Can you work these out from the model? Positions are in its coordinate system, mm. Face numbers are marked on the shaded views. A direction names the side the tool comes from. Give positions to 0.01 mm unless a question says otherwise; leave off trailing zeros. Loops run counter-clockwise (first coordinate to the right, second up) from the corner with the lowest first, then second, coordinate; pieces in that order, holes last. Notation, with made-up numbers: (47, 57) - (89, 57) arc R12 cw to (89, 72) - close; hole circle Ø5 at (-10.75, 67). An arc over 180 degrees is marked (long way). Answer as a JSON object with one key per item and string values.
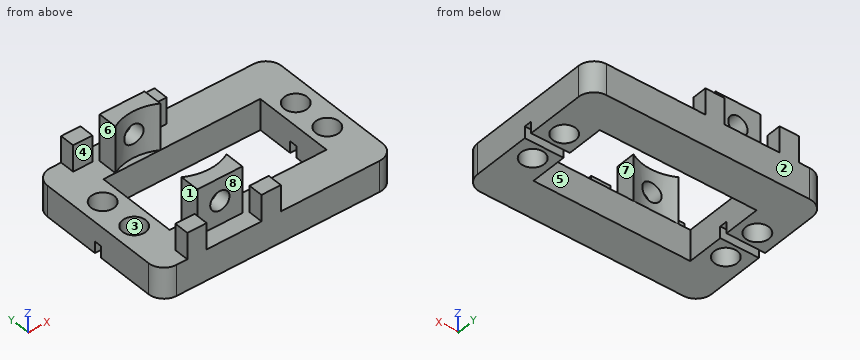
```python
from build123d import *

# Parameters (mm, degrees)
SKETCH_W        = 60.6
SKETCH_H        = 40
SKETCH_R        = 3
SKETCH_W_2      = 40.6
SKETCH_H_2      = 21
PAD_DEPTH       = 10
SKETCH001_W     = 60.6
SKETCH001_H     = 2
POCKET_DEPTH    = 3
PAD001_DEPTH    = 10
SKETCH003_R     = 2.5
POCKET001_DEPTH = 35.501
SKETCH004_W     = 5
SKETCH004_H     = 3.8
PAD002_DEPTH    = 4.8
PAD002_FACE4_R  = 3
POCKET002_DEPTH = 2
POCKET003_DEPTH = 2
POCKET004_DEPTH = 2
FILLET_R        = 4


with BuildPart() as part:
    # Sketch → Pad (new body)
    with BuildSketch(Plane.XY):
        with Locations((11.4, 0)):
            Rectangle(SKETCH_W, SKETCH_H)
        with Locations((-13.6, 5)):
            Circle(SKETCH_R, mode=Mode.SUBTRACT)
        with Locations((-13.6, -5)):
            Circle(SKETCH_R, mode=Mode.SUBTRACT)
        with Locations((36.4, 5)):
            Circle(SKETCH_R, mode=Mode.SUBTRACT)
        with Locations((36.4, -5)):
            Circle(SKETCH_R, mode=Mode.SUBTRACT)
        with Locations((11.4, 0)):
            Rectangle(SKETCH_W_2, SKETCH_H_2, mode=Mode.SUBTRACT)
    extrude(amount=PAD_DEPTH)

    # Sketch001 (on DatumPlane) → Pocket (cut)
    with BuildSketch(Plane.XY):
        with Locations((11.4, 0)):
            Rectangle(SKETCH001_W, SKETCH001_H)
    extrude(amount=POCKET_DEPTH, mode=Mode.SUBTRACT)

    # Sketch002 (on Face5 of Pocket) → Pad001 (join)
    with BuildSketch(Plane.XY.offset(10)):
        with BuildLine():
            Line((-5.809475, 15.5), (5.809475, 15.5))
            Line((5.809475, 15.5), (5.809475, 10.5))
            ThreePointArc((5.809475, 10.5), (0, 12), (-5.809475, 10.5))
            Line((-5.809475, 10.5), (-5.809475, 15.5))
        make_face()
        with BuildLine():
            Line((5.809475, -10.5), (5.809475, -15.5))
            Line((5.809475, -15.5), (-5.809475, -15.5))
            Line((-5.809475, -15.5), (-5.809475, -10.5))
            ThreePointArc((-5.809475, -10.5), (0, -12), (5.809475, -10.5))
        make_face()
    extrude(amount=PAD001_DEPTH)

    # Sketch003 (on Face23 of Pad001) → Pocket001 (cut, through all)
    with BuildSketch(Plane.XZ.offset(15.5)):
        with Locations((0, 14.1)):
            Circle(SKETCH003_R)
    extrude(amount=-POCKET001_DEPTH, mode=Mode.SUBTRACT)

    # Sketch004 (on Face5 of Pocket001) → Pad002 (join)
    with BuildSketch(Plane.XY.offset(10)):
        with Locations((9.6, 18.1)):
            Rectangle(SKETCH004_W, SKETCH004_H)
        with Locations((-9.6, 18.1)):
            Rectangle(SKETCH004_W, SKETCH004_H)
        with Locations((-9.6, -18.1)):
            Rectangle(SKETCH004_W, SKETCH004_H)
        with Locations((9.6, -18.1)):
            Rectangle(SKETCH004_W, SKETCH004_H)
    extrude(amount=PAD002_DEPTH)

    # Pad002 Face4 → Pocket002 (cut)
    with BuildSketch(Plane(origin=(13.130462, 0, 10), x_dir=(0, 1, 0), z_dir=(0, 0, 1))):
        Polygon((20, 25.230462), (20, 32.030462), (-20, 32.030462), (-20, 25.230462), (-16.2, 25.230462), (-16.2, 20.230462), (-20, 20.230462), (-20, 6.030462), (-16.2, 6.030462), (-16.2, 1.030462), (-20, 1.030462), (-20, -28.569538), (20, -28.569538), (20, 1.030462), (16.2, 1.030462), (16.2, 6.030462), (20, 6.030462), (20, 20.230462), (16.2, 20.230462), (16.2, 25.230462), align=None)
        with Locations((-5, 26.730462)):
            Circle(PAD002_FACE4_R, mode=Mode.SUBTRACT)
        with Locations((-5, -23.269538)):
            Circle(PAD002_FACE4_R, mode=Mode.SUBTRACT)
        with Locations((5, 26.730462)):
            Circle(PAD002_FACE4_R, mode=Mode.SUBTRACT)
        Polygon((-10.5, 22.030462), (10.5, 22.030462), (10.5, 18.939937), (15.5, 18.939937), (15.5, 7.320987), (10.5, 7.320987), (10.5, -18.569538), (-10.5, -18.569538), (-10.5, 7.320987), (-15.5, 7.320987), (-15.5, 18.939937), (-10.5, 18.939937), align=None, mode=Mode.SUBTRACT)
        with Locations((5, -23.269538)):
            Circle(PAD002_FACE4_R, mode=Mode.SUBTRACT)
    extrude(amount=-POCKET002_DEPTH, mode=Mode.SUBTRACT)

    # Pocket002 Face25 → Pocket003 (cut)
    with BuildSketch(Plane(origin=(0, 11.103335, 10), x_dir=(0, 1, 0), z_dir=(0, 0, 1))):
        with BuildLine():
            ThreePointArc((-0.603335, -5.809475), (0.896665, 0), (-0.603335, 5.809475))
            Line((-0.603335, 5.809475), (-0.603335, -5.809475))
        make_face()
    extrude(amount=-POCKET003_DEPTH, mode=Mode.SUBTRACT)

    # Pocket003 Face45 → Pocket004 (cut)
    with BuildSketch(Plane(origin=(0, -11.103335, 10), x_dir=(0, 1, 0), z_dir=(0, 0, 1))):
        with BuildLine():
            Line((0.603335, -5.809475), (0.603335, 5.809475))
            ThreePointArc((0.603335, 5.809475), (-0.896665, 0), (0.603335, -5.809475))
        make_face()
    extrude(amount=-POCKET004_DEPTH, mode=Mode.SUBTRACT)

    # Fillet
    fillet_edges = [part.edges().sort_by_distance(p)[0] for p in [
        (-18.9, -20, 4),
        (-18.9, 20, 4),
        (41.7, -20, 4),
        (41.7, 20, 4),
    ]]
    fillet(fillet_edges, radius=FILLET_R)


solid = part.part
```
1) Imagine slicing it at D-D on x = 0. Write out the boundary of the cut face in (y, z).
Check sheet entries:
{"outline": "(-20, 0) - (-10.5, 0) - (-10.5, 8) - (-12, 8) - (-12, 11.6) - (-15.5, 11.6) - (-15.5, 8) - (-20, 8) - close; (-15.5, 16.6) - (-12, 16.6) - (-12, 20) - (-15.5, 20) - close; (10.5, 0) - (20, 0) - (20, 8) - (15.5, 8) - (15.5, 11.6) - (12, 11.6) - (12, 8) - (10.5, 8) - close; (12, 16.6) - (15.5, 16.6) - (15.5, 20) - (12, 20) - close"}
2) If we mould it in two halves opening along X, with no side actions, what happens to the marked faces 1, 2 and 3? For each: released by +X, released by -X, zero draft, split by the parting line, or undercut.
Check sheet entries:
{"face 1": "released by -X", "face 2": "zero draft", "face 3": "undercut"}
3) I need wall thicknesses on L1, parallel to Y at x = -13.6, z = 5.25; L2, parallel to Z at x = 0, y = 13.65; L3, parallel to Y at x = 30, z = 5.5. Which ranges of each line are inside material? Lowest first, please.
Check sheet entries:
{"L1": "-20 to -8, -2 to 2, 8 to 20", "L2": "0 to 11.6, 16.6 to 20", "L3": "-20 to -10.5, 10.5 to 20"}
4) I'm going to push flat-ended pins straight in: P1, Ø3.5, axis at x = 36.4, y = -5, coming from the +Z side (3 decimals); P2, Ø1.1, axis at y = -17.5, z = 12.5, coming from the -X side; P3, Ø4, axis at x = 17, y = 9, coming from the +Z side; P4, Ø3, axis at y = -19, z = 12.5, coming from the +X side. Where does each tip first touch, or does it pass through?
Check sheet entries:
{"P1": "through", "P2": "x = -12.1", "P3": "z = 8", "P4": "x = 12.1"}
5) Which directions (+Z, -Z, +X, -X, +Y, -Y) give clear straight access to the entire face, cutting with the end or side of a thin tool? Please do the marked faces 4, 5, 6, 7 and 8.
Check sheet entries:
{"face 4": "+Z, +X, -X", "face 5": "+Z, -Z", "face 6": "+Z, -X, +Y, -Y", "face 7": "+Z, +X, +Y, -Y", "face 8": "+Z, +X, -X, -Y"}
6) Imagine slicing it at C-C on y = -5. Write out the boundary of the cut face in (x, z).
Check sheet entries:
{"outline": "(-18.9, 0) - (-16.6, 0) - (-16.6, 8) - (-18.9, 8) - close; (-10.6, 0) - (-8.9, 0) - (-8.9, 8) - (-10.6, 8) - close; (31.7, 0) - (33.4, 0) - (33.4, 8) - (31.7, 8) - close; (39.4, 0) - (41.7, 0) - (41.7, 8) - (39.4, 8) - close"}
7) Imagine slicing it at B-B on x = 24. Write out the boundary of the cut face in (y, z).
Check sheet entries:
{"outline": "(-20, 0) - (-10.5, 0) - (-10.5, 8) - (-20, 8) - close; (10.5, 0) - (20, 0) - (20, 8) - (10.5, 8) - close"}
8) Imagine slicing it at A-A on z = 14.1. Give the number of separate pieces and of enclosed holes in the cut face, and give its area (3 significant figures).
Check sheet entries:
{"separate pieces": "8", "enclosed holes": "0", "area": "133 mm2"}
